Study the drawing (mm; zero at the part's minimum x, y, z) and answer. A direction names the side the tool comes from. Coordinates: 2 decimals unless noted, no trailing zeros. Loops run counter-clockwise (first coordinate to the right, second up) from the corner with the lowest first, then second, coordinate; pieces in that order, holes last. Notation, with made-up numbers: (65.5, 76) - (82.5, 76) arc R14 ccw to (82.5, 87) - close; hole circle Ø5 at (24, 11). An arc over 180 degrees is marked (long way). Use one line per item in the form item = value. Start each with the question number.
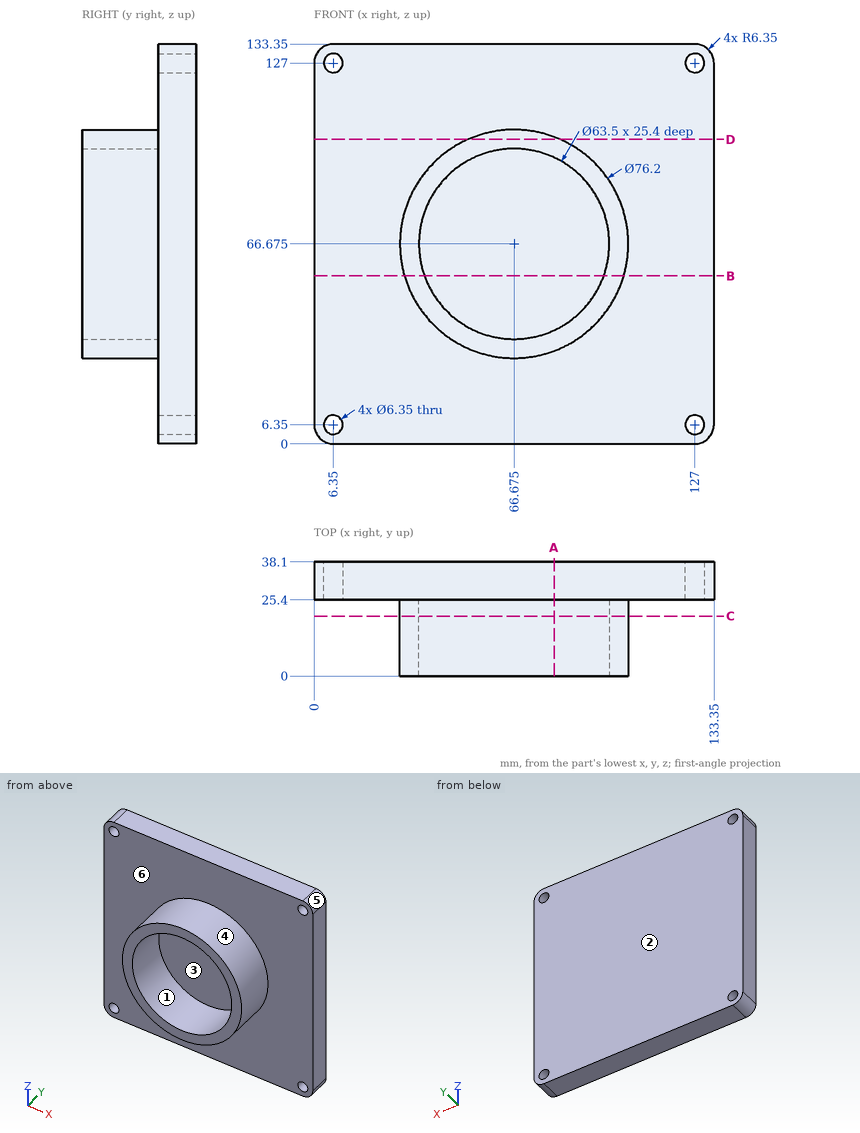
(1) For the marked faces 1 and 2, determine the directions among +Z, -Z, +X, -X, +Y, -Y from which every point of the face is accessible in a straight line to the end or side of a thin tool.
(2) A cutting plane is placed at B-B (z = 56). Determine the outline of the cut face in (x, y).
(3) A cutting plane is placed at D-D (z = 101.5). Determine the outline of the cut face in (x, y), then the cut area to 3 significant figures.
(4) A cutting plane is placed at A-A (x = 80). Determine the outline of the cut face in (y, z), then the cut area to 3 significant figures.
(5) Find the intervals of material crossed by probe 1 along Z at (x, y) = (127, 34) (3 decimals); probe 2 along Z at (x, y) = (125, 31), in increasing order. Write a range as from..to.
(6) Determine the mould class of the marked faces 3, 4, 5 and 6 for opening direction X: +X half, -X half, draft (parallel to the pull), parting line (faces both ways), or undercut.
(7) Each of these flat-tipped pins is pushed along its axis until it touches: pin 1 Ø6 at (x, y) = (61, 13) entering from -Z; pin 2 Ø19 at (x, z) = (70.5, 64.5) entering from -Y. Where does it stop, or does it pass through?
(8) A cutting plane is placed at C-C (y = 20). Determine the outline of the cut face in (x, z) (3 decimals).
Evaluation:
q1.face_1 = -Y
q1.face_2 = +Z, -Z, +X, -X, +Y
q2.outline = (0, 25.4) - (30.1, 25.4) - (30.1, 0) - (36.77, 0) - (36.77, 25.4) - (96.58, 25.4) - (96.58, 0) - (103.25, 0) - (103.25, 25.4) - (133.35, 25.4) - (133.35, 38.1) - (0, 38.1) - close
q3.outline = (0, 25.4) - (51.22, 25.4) - (51.22, 0) - (82.13, 0) - (82.13, 25.4) - (133.35, 25.4) - (133.35, 38.1) - (0, 38.1) - close
q3.area = 2,480 mm^2
q4.outline = (0, 30.98) - (25.4, 30.98) - (25.4, 0) - (38.1, 0) - (38.1, 133.35) - (25.4, 133.35) - (25.4, 102.37) - (0, 102.37) - (0, 95.49) - (25.4, 95.49) - (25.4, 37.86) - (0, 37.86) - close
q4.area = 2,040 mm^2
q5.probe_1 = 0..3.175, 9.525..123.825, 130.175..133.35
q5.probe_2 = 0..3.88, 8.82..124.53, 129.47..133.35
q6.face_3 = undercut
q6.face_4 = parting line
q6.face_5 = +X half
q6.face_6 = draft
q7.pin_1 = 28.67
q7.pin_2 = 25.4
q8.outline = circle Ø76.2 at (66.675, 66.675); hole circle Ø63.5 at (66.675, 66.675)
